The listing builds one solid part. Answer for the finished solid, in the listing's coordinates (mm). A direction names the side the tool comes from. Coordinates: 2 decimals unless noted, no trailing zeros. Loops run counter-clockwise (first coordinate to the right, second up) from the corner with the lowest first, then second, coordinate; pieces in that order, holes last. Notation, with made-up numbers: M 26.25,20.5 L 33.25,20.5 A21 cw 33.25,31.5 Z; hole C -27.5,69.5 d4. An arc over 180 degrees is marked long. Answer as a JSON object with one key per item and string values. Group by question number.
1. A cutting plane is placed at D-D on x = -13. Give the vertices of the cut face in (y, z), and give its area (3 significant figures).
2. Determine the mould class of faces 4 (the face through (29.445, 1.775, 20.661)), 5 (the face through (27.915, 1.775, -31.084)), 6 (the face through (-33.217, 1.825, 33.147)), 7 (the face through (34.5, 2, 0)) for opening direction Z: released by +Z, released by -Z, zero draft, split by the parting line, or undercut.
3. A cutting plane is placed at A-A on z = -25. Give the vertices of the cut face in (x, y).
4. Given pin 1 (1.7 mm diameter, centred on x = 30, z = 0, fed in from +Y), flat-ended and moving along its own axis, determine where the tip first touches the part or whether it passes through.
5. A cutting plane is placed at B-B on x = -4.5. Give the vertices of the cut face in (y, z).
6. Straight lines are drawn through the part: L1, parallel to X at y = 2.6, z = 0; L2, parallel to X at y = 1.6, z = 22; L3, parallel to X at y = 2.35, z = -22. For each, find the intervals that lie inside material, in ascending order.
7. For faces 1 (the face through (26.5, 2, 30)), 2 (the face through (-31.416, 1.775, 0.314)), 3 (the face through (0, 2, -17.5)), determine the directions among +Z, -Z, +X, -X, +Y, -Y from which every point of the face is accessible in a straight line to the end or side of a thin tool.
8. A cutting plane is placed at C-C on y = 2.45. State how many separate pieces and enclosed holes the cut face has, and give its area (3 significant figures).
from build123d import *

# Parameters (mm, degrees)
SKETCH1_W           = 70
SKETCH1_H           = 70
BOSS_EXTRUDE1_DEPTH = 3.6
SKETCH2_W           = 87.76827376
SKETCH2_H           = 85.716468358
CUT_EXTRUDE1_DEPTH  = 10
SKETCH4_R           = 2.35
SKETCH4_R_2         = 1.45
SKETCH4_R_3         = 9.2
CUT_EXTRUDE2_DEPTH  = 10


with BuildPart() as part:
    # Sketch1 → Boss-Extrude1 (new body)
    with BuildSketch(Plane(origin=(0, 0, 0), x_dir=(1, 0, 0), z_dir=(0, 1, 0))):
        Rectangle(SKETCH1_W, SKETCH1_H)
    extrude(amount=BOSS_EXTRUDE1_DEPTH)

    # Sketch2 → Cut-Extrude1 (cut)
    with BuildSketch(Plane(origin=(0, 3.6, 0), x_dir=(1, 0, 0), z_dir=(0, 1, 0))):
        Rectangle(SKETCH2_W, SKETCH2_H)
        with BuildLine():
            Line((30, 34.5), (28, 34.5))
            ThreePointArc((28, 34.5), (26.939339828, 34.060660172), (26.5, 33))
            Line((26.5, 33), (26.5, 20))
            ThreePointArc((26.5, 20), (25.767766953, 18.232233047), (24, 17.5))
            Line((24, 17.5), (-24, 17.5))
            ThreePointArc((-24, 17.5), (-25.767766953, 18.232233047), (-26.5, 20))
            Line((-26.5, 20), (-26.5, 33))
            ThreePointArc((-26.5, 33), (-26.939339828, 34.060660172), (-28, 34.5))
            Line((-28, 34.5), (-30, 34.5))
            ThreePointArc((-30, 34.5), (-33.181980515, 33.181980515), (-34.5, 30))
            Line((-34.5, 30), (-34.5, -30))
            ThreePointArc((-34.5, -30), (-33.181980515, -33.181980515), (-30, -34.5))
            Line((-30, -34.5), (-28, -34.5))
            ThreePointArc((-28, -34.5), (-26.939339828, -34.060660172), (-26.5, -33))
            Line((-26.5, -33), (-26.5, -27))
            ThreePointArc((-26.5, -27), (-25.767766953, -25.232233047), (-24, -24.5))
            Line((-24, -24.5), (24, -24.5))
            ThreePointArc((24, -24.5), (25.767766953, -25.232233047), (26.5, -27))
            Line((26.5, -27), (26.5, -33))
            ThreePointArc((26.5, -33), (26.939339828, -34.060660172), (28, -34.5))
            Line((28, -34.5), (30, -34.5))
            ThreePointArc((30, -34.5), (33.181980515, -33.181980515), (34.5, -30))
            Line((34.5, -30), (34.5, 30))
            ThreePointArc((34.5, 30), (33.181980515, 33.181980515), (30, 34.5))
        make_face(mode=Mode.SUBTRACT)
    extrude(amount=-CUT_EXTRUDE1_DEPTH, mode=Mode.SUBTRACT)

    # Sketch4 → Cut-Extrude2 (cut)
    with BuildSketch(Plane.XZ):
        with Locations(Location((30, -30, 0), (0, 0, 270))):
            Circle(SKETCH4_R)
        with Locations(Location((30, -22, 0), (0, 0, 270))):
            Circle(SKETCH4_R_2)
        with Locations(Location((30, 0, 0), (0, 0, 270))):
            Circle(SKETCH4_R_2)
        with Locations(Location((30, 22, 0), (0, 0, 270))):
            Circle(SKETCH4_R_2)
        with Locations(Location((30, 30, 0), (0, 0, 270))):
            Circle(SKETCH4_R)
        with Locations(Location((-30, -30, 0), (0, 0, 270))):
            Circle(SKETCH4_R)
        with Locations(Location((-30, -22, 0), (0, 0, 270))):
            Circle(SKETCH4_R_2)
        with Locations(Location((0, 0, 0), (0, 0, 270))):
            Circle(SKETCH4_R_3)
        with Locations(Location((-30, 0, 0), (0, 0, 270))):
            Circle(SKETCH4_R_2)
        with Locations(Location((-30, 22, 0), (0, 0, 270))):
            Circle(SKETCH4_R_2)
        with Locations(Location((-30, 30, 0), (0, 0, 270))):
            Circle(SKETCH4_R)
    extrude(amount=-CUT_EXTRUDE2_DEPTH, mode=Mode.SUBTRACT)


solid = part.part
From the geometry:
{
 "1": {"outline": "M 0,-17.5 L 3.6,-17.5 L 3.6,24.5 L 0,24.5 Z", "area": "151 mm²"},
 "2": {"face 4": "undercut", "face 5": "undercut", "face 6": "released by +Z", "face 7": "zero draft"},
 "3": {"outline": "M -34.5,0 L -26.5,0 L -26.5,3.6 L -34.5,3.6 Z; M 26.5,0 L 34.5,0 L 34.5,3.6 L 26.5,3.6 Z"},
 "4": {"pin 1": "passes through"},
 "5": {"outline": "M 0,-17.5 L 3.6,-17.5 L 3.6,-8.02 L 0,-8.02 Z; M 0,8.02 L 3.6,8.02 L 3.6,24.5 L 0,24.5 Z"},
 "6": {"L1": "x = -34.5 to -31.45, -28.55 to -9.2, 9.2 to 28.55, 31.45 to 34.5", "L2": "x = -34.5 to -31.45, -28.55 to 28.55, 31.45 to 34.5", "L3": "x = -34.5 to -31.45, -28.55 to -26.5, 26.5 to 28.55, 31.45 to 34.5"},
 "7": {"face 1": "+Z, +Y, -Y", "face 2": "+Y, -Y", "face 3": "-Z, +Y, -Y"},
 "8": {"separate pieces": "1", "enclosed holes": "11", "area": "2,940 mm²"}
}
